from build123d import *

# Parameters (mm, degrees)
F1_DEPTH = 10


with BuildPart() as f1:
    # F0 (on Front) → F1 (new body)
    with BuildSketch(Plane.XZ):
        with BuildLine():
            ThreePointArc((13.428571, 187.091175), (13.660124, 188.595138), (14.333333, 189.959803))
            ThreePointArc((14.333333, 189.959803), (0, 217.5), (-14.333333, 189.959803))
            ThreePointArc((-14.333333, 189.959803), (-13.660124, 188.595138), (-13.428571, 187.091175))
            Line((-13.428571, 187.091175), (-13.428571, 12.908825))
            ThreePointArc((-13.428571, 12.908825), (-13.660124, 11.404862), (-14.333333, 10.040197))
            ThreePointArc((-14.333333, 10.040197), (0, -17.5), (14.333333, 10.040197))
            ThreePointArc((14.333333, 10.040197), (13.660124, 11.404862), (13.428571, 12.908825))
            Line((13.428571, 12.908825), (13.428571, 187.091175))
        make_face()
        with BuildLine():
            ThreePointArc((0, 10), (7.071068, 7.071068), (10, 0))
            ThreePointArc((10, 0), (-7.071068, -7.071068), (0, 10))
        make_face(mode=Mode.SUBTRACT)
        with BuildLine():
            ThreePointArc((10, 200), (7.071068, 192.928932), (0, 190))
            ThreePointArc((0, 190), (-7.071068, 207.071068), (10, 200))
        make_face(mode=Mode.SUBTRACT)
    extrude(amount=F1_DEPTH)


solid = f1.part
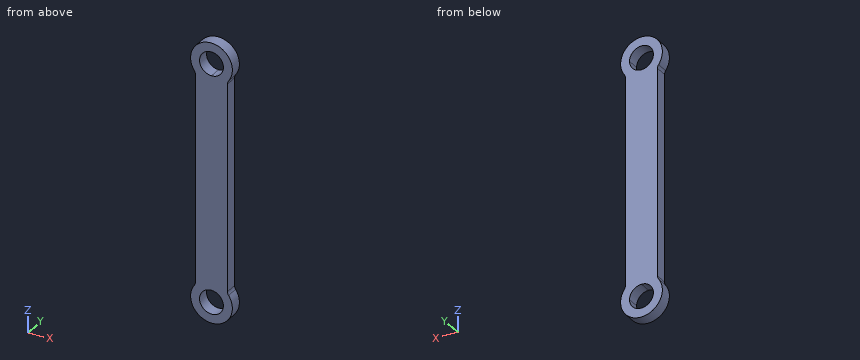
Can you work these out from the model? Positions are in its coordinate system, mm. Round coordinates to 2 decimals unless told otherwise and drop trailing zeros. Loops run counter-clockwise (first coordinate to the right, second up) from the corner with the lowest first, then second, coordinate; pieces in that order, holes last. Notation, with made-up numbers: (65, 11) - (86, 11) arc R14 cw to (86, 19) - close; hole circle Ø8 at (69.25, -9). An arc over 180 degrees is marked (long way). Use CSV: the item, a comma, the result in double quotes. Start each with the question number.
1) If we section it at A-A on y = -3.75: Write out the boundary of the cut face in (x, z), plus the area to 3 significant figures.
2) If we section it at D-D on x = -4: Write out the boundary of the cut face in (y, z), plus the area to 3 significant figures.
3) If we section it at C-C on z = 26: Write out the boundary of the cut face in (x, y), plus the area to 3 significant figures.
4) If we section it at B-B on x = 7.5: Write out the boundary of the cut face in (y, z), plus the area to 3 significant figures.
5) For pin 1 Ø5 at (y, z) = (-4, 73) entering from -X; pin 2 Ø3 at (y, z) = (-4.5, 90) entering from +X; pin 3 Ø1.5 at (x, y) = (-10.5, -3.5) entering from -Z, each with a flat end and sliding along its axis, tell me the tip position at first contact or that it passes through.
6) Please list where these lines run through material, in increasing order: probe 1 along Z at (x, y) = (-1, -3.5); probe 2 along Z at (x, y) = (-16, -2.5); probe 3 along X at (y, z) = (-6.75, 134). Write a range as [from, to].
Geometry results:
1,outline,"(-14.33, 10.04) arc R17.5 ccw (long way) to (14.33, 10.04) arc R5 cw to (13.43, 12.91) - (13.43, 187.09) arc R5 cw to (14.33, 189.96) arc R17.5 ccw (long way) to (-14.33, 189.96) arc R5 cw to (-13.43, 187.09) - (-13.43, 12.91) arc R5 cw to start; hole circle Ø20 at (0, 0); hole circle Ø20 at (0, 200)"
1,area,"5,830 mm2"
2,outline,"(-10, -17.04) - (0, -17.04) - (0, -9.17) - (-10, -9.17) - close; (-10, 9.17) - (0, 9.17) - (0, 190.83) - (-10, 190.83) - close; (-10, 209.17) - (0, 209.17) - (0, 217.04) - (-10, 217.04) - close"
2,area,"1,970 mm2"
3,outline,"(-13.43, -10) - (13.43, -10) - (13.43, 0) - (-13.43, 0) - close"
3,area,"269 mm2"
4,outline,"(-10, -15.81) - (0, -15.81) - (0, -6.61) - (-10, -6.61) - close; (-10, 6.61) - (0, 6.61) - (0, 193.39) - (-10, 193.39) - close; (-10, 206.61) - (0, 206.61) - (0, 215.81) - (-10, 215.81) - close"
4,area,"2,050 mm2"
5,pin 1,"stops at x = -13.43"
5,pin 2,"stops at x = 13.43"
5,pin 3,"stops at z = -14.53"
6,probe 1,"z = [-17.47, -9.95], [9.95, 190.05], [209.95, 217.47]"
6,probe 2,"z = [-7.09, 7.09], [192.91, 207.09]"
6,probe 3,"x = [-13.43, 13.43]"
